```python
from build123d import *

# Parameters (mm, degrees)
SKETCH1_W            = 170
SKETCH1_H            = 90
BOSS_EXTRUDE1_DEPTH  = 80
SKETCH3_W            = 170
SKETCH3_H            = 80
BOSS_EXTRUDE3_DEPTH  = 30
SKETCH5_W            = 155
SKETCH5_H            = 70
CUT_EXTRUDE3_DEPTH   = 110
SKETCH4_W            = 155
SKETCH4_H            = 10
CUT_EXTRUDE4_DEPTH   = 75
SKETCH6_W            = 1.5
SKETCH6_H            = 35
BOSS_EXTRUDE9_DEPTH  = 15
SKETCH7_W            = 152
SKETCH7_H            = 3.5
BOSS_EXTRUDE10_DEPTH = 5
SKETCH10_W           = 170
SKETCH10_H           = 80
SKETCH10_W_2         = 155
SKETCH10_H_2         = 70
BOSS_EXTRUDE13_DEPTH = 10
CUT_EXTRUDE5_DEPTH   = 81
SKETCH14_W           = 5
SKETCH14_H           = 60
CUT_EXTRUDE6_DEPTH   = 171


with BuildPart() as part:
    # Sketch1 → Boss-Extrude1 (new body)
    with BuildSketch(Plane(origin=(0, 0, 0), x_dir=(1, 0, 0), z_dir=(0, 1, 0))):
        Rectangle(SKETCH1_W, SKETCH1_H)
    extrude(amount=BOSS_EXTRUDE1_DEPTH)

    # Sketch3 → Boss-Extrude3 (add)
    with BuildSketch(Plane.XY.offset(45)):
        with Locations((0, 40)):
            Rectangle(SKETCH3_W, SKETCH3_H)
    extrude(amount=BOSS_EXTRUDE3_DEPTH)

    # Sketch5 → Cut-Extrude3 (cut)
    with BuildSketch(Plane.XY.offset(75)):
        with Locations((0, 40)):
            Rectangle(SKETCH5_W, SKETCH5_H)
    extrude(amount=-CUT_EXTRUDE3_DEPTH, mode=Mode.SUBTRACT)

    # Sketch4 → Cut-Extrude4 (cut)
    with BuildSketch(Plane(origin=(0, 80, 0), x_dir=(1, 0, 0), z_dir=(0, 1, 0))):
        with Locations((0, 30)):
            Rectangle(SKETCH4_W, SKETCH4_H)
    extrude(amount=-CUT_EXTRUDE4_DEPTH, mode=Mode.SUBTRACT)

    # Sketch6 → Boss-Extrude9 (add)
    with BuildSketch(Plane.XY.offset(-35)):
        with Locations((76.75, 22.5)):
            Rectangle(SKETCH6_W, SKETCH6_H)
        with Locations((-76.75, 22.5)):
            Rectangle(SKETCH6_W, SKETCH6_H)
    extrude(amount=BOSS_EXTRUDE9_DEPTH)

    # Sketch7 → Boss-Extrude10 (add)
    with BuildSketch(Plane(origin=(0, 5, 0), x_dir=(1, 0, 0), z_dir=(0, 1, 0))):
        with Locations((0, 21.25)):
            Rectangle(SKETCH7_W, SKETCH7_H)
    extrude(amount=BOSS_EXTRUDE10_DEPTH)

    # Sketch10 → Boss-Extrude13 (add)
    with BuildSketch(Plane.XY.offset(75)):
        with Locations((0, 40)):
            Rectangle(SKETCH10_W, SKETCH10_H)
        with Locations((0, 40)):
            Rectangle(SKETCH10_W_2, SKETCH10_H_2, mode=Mode.SUBTRACT)
    extrude(amount=BOSS_EXTRUDE13_DEPTH)

    # Sketch11 → Cut-Extrude5 (cut, through all)
    with BuildSketch(Plane(origin=(0, 80, 0), x_dir=(1, 0, 0), z_dir=(0, 1, 0))):
        with BuildLine():
            Line((77.5, -85), (-77.5, -85))
            ThreePointArc((-77.5, -85), (0, -76.559027761), (77.5, -85))
        make_face()
    extrude(amount=-CUT_EXTRUDE5_DEPTH, mode=Mode.SUBTRACT)

    # Sketch14 → Cut-Extrude6 (cut, through all)
    with BuildSketch(Plane(origin=(85, 0, 0), x_dir=(0, 0, -1), z_dir=(1, 0, 0))):
        with Locations((40.5, 40)):
            Rectangle(SKETCH14_W, SKETCH14_H)
    extrude(amount=-CUT_EXTRUDE6_DEPTH, mode=Mode.SUBTRACT)


solid = part.part
```
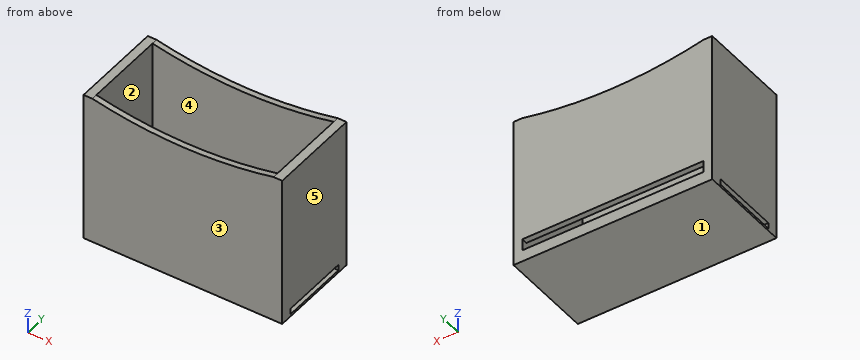
Work out the finished part from the listing and answer in its coordinate system (mm). Face numbers are marked on the shaded views. A direction names the side the tool comes from. Round coordinates to 2 decimals unless told otherwise and drop trailing zeros. Write each loop counter-clockwise with the first axis right and the second up, starting at its lowest first coordinate (ties: lowest second). Pieces come first, ordered by that corner, then holes. Notation, with made-up numbers: (22, -6) -> (57, -6) arc R24 ccw to (57, 7) -> close; hole circle Ø3 at (30, 36). An arc over 180 degrees is marked (long way). Write each question's results on one line, items separated by ' | '.
1) For a pull along Y with two mould halves and no side action, classify the marked faces 1, 2 and 3 as +Y half, -Y half, draft (parallel to the pull), parting line (faces both ways), or undercut.
Findings:
face 1: draft | face 2: undercut | face 3: -Y half
2) The part is cut by section B-B (x = 54.5). Write down the section's boundary in (y, z).
Findings:
outline: (0, -45) -> (80, -45) -> (80, -35) -> (5, -35) -> (5, -23) -> (10, -23) -> (10, -19.5) -> (5, -19.5) -> (5, 80.71) -> (0, 80.71) -> close; (75, -25) -> (80, -25) -> (80, 80.71) -> (75, 80.71) -> close; hole (10, -43) -> (70, -43) -> (70, -38) -> (10, -38) -> close
3) The part is cut by section A-A (y = 56.5). Write down the section's boundary in (x, z).
Findings:
outline: (-85, -45) -> (85, -45) -> (85, -43) -> (-85, -43) -> close; (-85, -38) -> (85, -38) -> (85, 85) -> (77.5, 85) -> (77.5, -35) -> (-77.5, -35) -> (-77.5, 85) -> (-85, 85) -> close
4) The part is cut by section C-C (z = 22). Write down the section's boundary in (x, y).
Findings:
outline: (-85, 0) -> (85, 0) -> (85, 80) -> (-85, 80) -> close; hole (-77.5, 5) -> (77.5, 5) -> (77.5, 75) -> (-77.5, 75) -> close
5) Flat-ended cylindrical pins translate along their axes: pin 1 (2.5 mm diameter, centred on x = 33, y = 8.5, fed in from +Z); pin 2 (18 mm diameter, centred on x = -14, y = 40, fed in from +Z); pin 3 (1.2 mm diameter, centred on x = -76.5, y = 30.5, fed in from +Z). Find the tip coordinate at first contact, or state that the pin passes through.
Findings:
pin 1: stops at z = -19.5 | pin 2: stops at z = -35 | pin 3: stops at z = -20
6) The part is cut by section D-D (y = 19). Write down the section's boundary in (x, z).
Findings:
outline: (-85, -45) -> (85, -45) -> (85, -43) -> (-85, -43) -> close; (-85, -38) -> (85, -38) -> (85, 85) -> (77.5, 85) -> (77.5, -20) -> (76, -20) -> (76, -35) -> (-76, -35) -> (-76, -20) -> (-77.5, -20) -> (-77.5, 85) -> (-85, 85) -> close
7) Consider line 1 along Y through (x, z) = (-3, 8); line 2 along Y through (x, z) = (-30, -21); line 3 along X through (y, z) = (6, 50.5). Determine where each line is inside the solid, lowest interval first. Write a range as [from, to].
Findings:
line 1: y = [0, 5], [75, 80] | line 2: y = [0, 10], [75, 80] | line 3: x = [-85, -77.5], [77.5, 85]
8) Which of the six approach directions +Z, -Z, +X, -X, +Y, -Y give full straight-line access (tool end or side, diameter ignored) to the marked faces 4 and 5?
Findings:
face 4: +Z | face 5: +Z, -Z, +X, +Y, -Y
